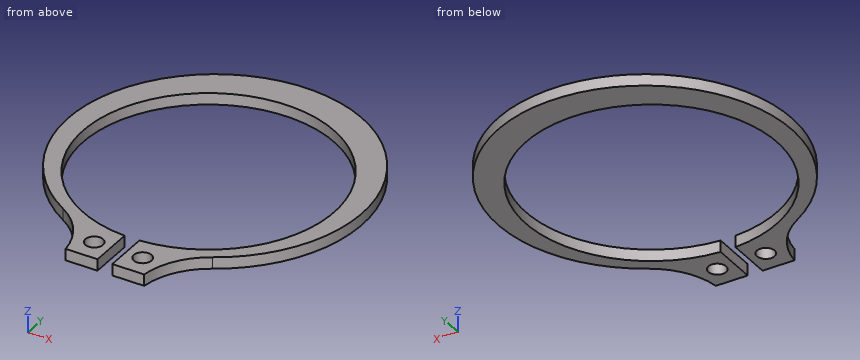
Autodesk Inventor part; units mm, degrees
ref_plane "YZ Plane" through (0, 0, 0) normal (1, 0, 0) x (0, 1, 0)
ref_plane "XZ Plane" through (0, 0, 0) normal (0, 1, 0) x (-1, 0, 0)
ref_plane "XY Plane" through (0, 0, 0) normal (0, 0, 1) x (1, 0, 0)
sketch "草图2" plane through (0, 0, 0) normal (0, 0, 1) x (1, 0, 0)
  line L0 (-0.8333, -19.1505) -> (-4.4333, -19.1505)
  line L1 (-0.8333, -14.1505) -> (-0.8333, -19.1505)
  arc A0 (0.8333, -14.1505) -> (-0.8333, -14.1505) centre (0, 0) ccw
  arc A1 (8.4124, -13.0815) -> (-8.4124, -13.0815) centre (0, 1.2) ccw
  line L2 (0, -19.4467) -> (0, 17.2703)
  line L3 (0.8333, -19.1505) -> (4.4333, -19.1505)
  line L4 (0.8333, -14.1505) -> (0.8333, -19.1505)
  arc A2 (-4.4333, -19.1505) -> (-8.4124, -13.0815) centre (-12.5763, -20.1505) ccw
  arc A3 (8.4124, -13.0815) -> (4.4333, -19.1505) centre (12.5763, -20.1505) ccw
  dimension "d15" = 1.2
  dimension "d28" = 28.35
  dimension "d32" = 3.6
  dimension "d34" = 5
  dimension "d35" = 1.6667
  dimension "d48" = 3.6
  dimension "d49" = 1
extrude "拉伸1" add sketch "草图2" against normal blind 1.3
sketch "草图3" plane through (0, 0, 0) normal (0, 0, 1) x (1, 0, 0)
  circle A0 centre (-2.7333, -16.6505) radius 1
  line L0 (-0.8333, -19.1505) -> (-4.4333, -19.1505)
  line L1 (0.8333, -19.1505) -> (0.8333, -14.1505)
  line L2 (4.4333, -19.1505) -> (0.8333, -19.1505)
  line L3 (0, -14.2014) -> (0, -8.6014)
  circle A1 centre (2.7333, -16.6505) radius 1
  dimension "d36" = 2
  dimension "d37" = 2.5
  dimension "d47" = 5.4667
extrude "拉伸2" cut sketch "草图3" against normal through all
equation "\"d15\" = 0.333333 * b"
equation "\"d28\" = g1"
equation "\"d32\" = b"
equation "\"d34\" = ParA"
equation "\"d35\" = 0.333333 * ParA"
equation "\"d48\" = 1.8 * Diam5"
equation "\"d49\" = 0.2 * ParA"
equation "\"d16\" = tt"
equation "\"d36\" = Diam5"
equation "\"d37\" = 0.5 * ParA"
equation "\"d47\" = 0.333333 * ParA + 1.9 * Diam5"
equation "\"g1\" = 28.35"
equation "\"ParA\" = 5"
equation "\"tt\" = 1.3"
equation "\"Diam5\" = 2"
equation "\"TEMPLATE\" = 1.2345"
properties part number "ANSI B 27.7M - 3AMI-30" material "钢，软"
Input: part model. Units: mm. Frame: model coordinates. Round coordinates to 2 decimals unless told otherwise and drop trailing zeros. Order: outer loops, then holes, each group sorted by start corner. A loop starts at its lowest first (then second) coordinate and runs counter-clockwise, first axis right, second up.
1. Pin query (flat end, axial travel): P1, Ø0.6, axis at y = -16, z = -0.5, coming from the +X side; P2, Ø2.5, axis at x = 2.73, y = -16.65, coming from the +Z side; P3, Ø1, axis at x = -7.5, y = 10.5, coming from the -Z side. Return the tip coordinate at first contact, or that it passes through.
The answers:
P1: stops at x = 5.68
P2: stops at z = 0
P3: passes through
2. Cut plane A-A, the plane x = 7.5. Output: boundary loops of the cut face in (y, z).
The answers:
outline: (-13.71, -1.3) - (-12.03, -1.3) - (-12.03, 0) - (-13.71, 0) - close; (12.03, -1.3) - (15.98, -1.3) - (15.98, 0) - (12.03, 0) - close
3. Material intervals for line 1 (Y direction, x = 3.5, z = -0.35); line 2 (Y direction, x = -2.5, z = -0.55); line 3 (Y direction, x = -0.5, z = -1.05), sorted ascending.
The answers:
line 1: y = -19.15 to -17.29, -16.01 to -13.74, 13.74 to 17.4
line 2: y = -19.15 to -17.62, -15.68 to -13.95, 13.95 to 17.59
line 3: y = 14.17 to 17.77
4. Cut plane D-D, the plane x = 0. Output: boundary loops of the cut face in (y, z), then the cut area to 3 significant figures.
The answers:
outline: (14.18, -1.3) - (17.77, -1.3) - (17.77, 0) - (14.18, 0) - close
area: 4.68 mm2
5. Cut plane B-B, the plane y = 1.2. Output: boundary loops of the cut face in (x, z), then the cut area to 3 significant figures.
The answers:
outline: (-16.57, -1.3) - (-14.12, -1.3) - (-14.12, 0) - (-16.57, 0) - close; (14.12, -1.3) - (16.57, -1.3) - (16.57, 0) - (14.12, 0) - close
area: 6.37 mm2
6. Cut plane C-C, the plane z = -0.3. Output: boundary loops of the cut face in (x, y).
The answers:
outline: (-8.41, -13.08) arc R8.2 cw to (-4.43, -19.15) - (-0.83, -19.15) - (-0.83, -14.15) arc R14.18 cw (long way) to (0.83, -14.15) - (0.83, -19.15) - (4.43, -19.15) arc R8.2 cw to (8.41, -13.08) arc R16.57 ccw (long way) to start; hole circle Ø2 at (-2.73, -16.65); hole circle Ø2 at (2.73, -16.65)
